```python
from build123d import *

# Parameters (mm, degrees)
F0_W     = 762
F0_H     = 609.6
F1_DEPTH = 30
F2_W     = 10
F2_H     = 594.36
F3_DEPTH = 596.9
F4_R     = 19.05
F5_DEPTH = 38.1


with BuildPart() as f1:
    # F0 (on Front) → F1 (new body)
    with BuildSketch(Plane.XZ):
        Rectangle(F0_W, F0_H)
    extrude(amount=F1_DEPTH)

    # F2 (on face) → F3 (cut)
    with BuildSketch(Plane(origin=(-381, 0, 0), x_dir=(0, -1, 0), z_dir=(-1, 0, 0))):
        with Locations((15, 0)):
            Rectangle(F2_W, F2_H)
    extrude(amount=-F3_DEPTH, mode=Mode.SUBTRACT)

    # F4 (on face) → F5 (join)
    with BuildSketch(Plane(origin=(0, 0, 0), x_dir=(-1, 0, 0), z_dir=(0, 1, 0))):
        with Locations((-330.2, 254)):
            Circle(F4_R)
        with Locations((330.2, 254)):
            Circle(F4_R)
        with Locations((330.2, -254)):
            Circle(F4_R)
        with Locations((-330.2, -254)):
            Circle(F4_R)
    extrude(amount=F5_DEPTH)


solid = f1.part
```
Input: part model. Units: mm. Frame: model coordinates. A direction names the side the tool comes from. Round coordinates to 2 decimals unless told otherwise and drop trailing zeros. Loops run counter-clockwise (first coordinate to the right, second up) from the corner with the lowest first, then second, coordinate; pieces in that order, holes last. Notation, with made-up numbers: (-29.5, 69.25) - (-5.5, 69.25) arc R25 cw to (-5.5, 85.25) - close; hole circle Ø10 at (4, 31). An arc over 180 degrees is marked (long way). One line per item, written item: value. Start each with the question number.
(1) Ray query, line 1 (Y direction, x = -258.5, z = -70.5); line 2 (X direction, y = -10.5, z = -49); line 3 (Z direction, x = 335, y = 4.5). Return the intervals inside material, ascending. Write a range as [from, to].
(2) Draft query along Z for faces 4 (the flat face through (-5, -15, -304.8)), 5 (the flat face through (381, -15, -4)), 6 (the cylindrical face through (-316.159, 18.783, -241.125)). Return one class per face: +Z half, -Z half, draft (parallel to the pull), parting line (faces both ways), or undercut.
(3) Contact query for a flat-ended pin moving along its axis: P1, Ø1.5, axis at x = 184.5, z = -20.5, coming from the +Y side. Output: stop coordinate, or through.
(4) Section A-A, the plane x = -330.2. Return loops of the section in (y, z), plus the area to 3 significant figures.
(5) Section B-B, the plane z = 254. Return loops of the section in (x, y).
(6) Access query for faces 1 (the cylindrical face through (319.959, 18.783, 270.063)), 2 (the flat face through (-330, 38.1, 254)), 3 (the flat face through (-87, -20, -4)). Directions: +Z, -Z, +X, -X, +Y, -Y. A direction counts if a zero-diameter tool reaches every point of the face in a straight line with its end or side. Return the directions, or none.
(7) Section C-C, the plane y = 28.5. Return loops of the section in (x, z), plus the area to 3 significant figures.
(8) Section D-D, the plane x = 330.2. Return loops of the section in (y, z), plus the area to 3 significant figures.
Results below:
1. line 1: [-30, -20], [-10, 0]
1. line 2: [215.9, 381]
1. line 3: [-272.44, -235.56], [235.56, 272.44]
2. face 4: -Z half
2. face 5: draft
2. face 6: undercut
3. P1: y = 0
4. outline: (-30, -304.8) - (0, -304.8) - (0, -273.05) - (38.1, -273.05) - (38.1, -234.95) - (0, -234.95) - (0, 234.95) - (38.1, 234.95) - (38.1, 273.05) - (0, 273.05) - (0, 304.8) - (-30, 304.8) - close; hole (-20, -297.18) - (-10, -297.18) - (-10, 297.18) - (-20, 297.18) - close
4. area: 15,200 mm^2
5. outline: (-381, -30) - (381, -30) - (381, 0) - (349.25, 0) - (349.25, 38.1) - (311.15, 38.1) - (311.15, 0) - (-311.15, 0) - (-311.15, 38.1) - (-349.25, 38.1) - (-349.25, 0) - (-381, 0) - (-381, -10) - (215.9, -10) - (215.9, -20) - (-381, -20) - close
6. face 1: +Y
6. face 2: +Z, -Z, +X, -X, +Y
6. face 3: -X
7. outline: circle Ø38.1 at (-330.2, -254); circle Ø38.1 at (-330.2, 254); circle Ø38.1 at (330.2, -254); circle Ø38.1 at (330.2, 254)
7. area: 4,560 mm^2
8. outline: (-30, -304.8) - (0, -304.8) - (0, -273.05) - (38.1, -273.05) - (38.1, -234.95) - (0, -234.95) - (0, 234.95) - (38.1, 234.95) - (38.1, 273.05) - (0, 273.05) - (0, 304.8) - (-30, 304.8) - close
8. area: 21,200 mm^2
